Could you check a few things on this model? Use its own coordinates, in mm. A direction names the side the tool comes from. Coordinates: 2 decimals unless noted, no trailing zeros. Loops run counter-clockwise (first coordinate to the right, second up) from the corner with the lowest first, then second, coordinate; pieces in that order, holes last.
from build123d import *

# Parameters (mm, degrees)
BOSS_EXTRUDE1_DEPTH = 60
SKETCH2_W           = 10
SKETCH2_H           = 50
CUT_EXTRUDE1_DEPTH  = 25
SKETCH3_W           = 10
SKETCH3_H           = 50
CUT_EXTRUDE2_DEPTH  = 25
FILLET1_R           = 2
SKETCH4_R           = 2
CUT_EXTRUDE3_DEPTH  = 25


with BuildPart() as part:
    # Sketch1 → Boss-Extrude1 (new body)
    with BuildSketch(Plane(origin=(0, 0, 0), x_dir=(1, 0, 0), z_dir=(0, 1, 0))):
        with BuildLine():
            Line((-4.271755912, 52.025339674), (24.498929667, 52.025339674))
            ThreePointArc((24.498929667, 52.025339674), (-8.501070333, 19.025339674), (24.498929667, -13.974660326))
            Line((24.498929667, -13.974660326), (-4.271755912, -13.974660326))
            Line((-4.271755912, -13.974660326), (-4.271755912, -77.974660326))
            Line((-4.271755912, -77.974660326), (-14.271755912, -77.974660326))
            Line((-14.271755912, -77.974660326), (-14.271755912, 52.025339674))
            Line((-14.271755912, 52.025339674), (-4.271755912, 52.025339674))
        make_face()
    extrude(amount=BOSS_EXTRUDE1_DEPTH)

    # Sketch2 → Cut-Extrude1 (cut)
    with BuildSketch(Plane(origin=(0, 60, 0), x_dir=(1, 0, 0), z_dir=(0, 1, 0))):
        with Locations((-9.271755912, -52.974660326)):
            Rectangle(SKETCH2_W, SKETCH2_H)
    extrude(amount=-CUT_EXTRUDE1_DEPTH, mode=Mode.SUBTRACT)

    # Sketch3 → Cut-Extrude2 (cut)
    with BuildSketch(Plane.XZ):
        with Locations((-9.271755912, 52.974660326)):
            Rectangle(SKETCH3_W, SKETCH3_H)
    extrude(amount=-CUT_EXTRUDE2_DEPTH, mode=Mode.SUBTRACT)

    # Fillet1
    fillet1_edges = [part.edges().sort_by_distance(p)[0] for p in [
        (24.498929667, 30, -52.025339674),
        (24.498929667, 30, 13.974660326),
    ]]
    fillet(fillet1_edges, radius=FILLET1_R)

    # Sketch4 → Cut-Extrude3 (cut)
    with BuildSketch(Plane(origin=(0, 35, 0), x_dir=(1, 0, 0), z_dir=(0, 1, 0))):
        with Locations((-9.271755912, -65.474660326)):
            Circle(SKETCH4_R)
    extrude(amount=-CUT_EXTRUDE3_DEPTH, mode=Mode.SUBTRACT)


solid = part.part
1) Imagine slicing it at C-C on z = -35. List the corners of the cut face in (x, y) for me.
2) Will these pins go through, and if not, where does the flat tip stop? pin 1 (8 mm diameter, centred on x = -10, y = 16.5, fed in from +Z); pin 2 (2.5 mm diameter, centred on x = -9.27, z = 65.47, fed in from +Y); pin 3 (5 mm diameter, centred on x = -11.5, z = 44.5, fed in from -Y); pin 4 (1.5 mm diameter, centred on x = 4.5, y = 19, fed in from +Z).
3) Imagine slicing it at B-B on z = 25.5. List the corners of the cut face in (x, y) for me, plus the area to 3 significant figures.
4) If I drill on L1, parallel to Y at x = -11.5, z = 37; L2, parallel to Z at x = 9.25, y = 4; L3, parallel to Z at x = -3, y = 26, over which ranges is the centre line in solid material (lowest first)?
5) For faces 1 (the flat face through (2, 30, 13.975)), 2 (the flat face through (-9, 48, 27.975)), 3 (the flat face through (-9, 25, 53)), which set-ups out of +Z, -Z, +X, -X, +Y, -Y let a thin tool reach every point of the face, with its end or its side?
6) We'd pull the mould along Z, two halves only. Please class faces 4 (the flat face through (-9, 12, 27.975)), 5 (the flat face through (-4.272, 28, 32)), 6 (the cylindrical face through (10.2, 30.42, 12.42)): released by +Z, released by -Z, zero draft, split by the parting line, or undercut.
7) Imagine slicing it at A-A on x = 0. List the corners of the cut face in (y, z) for me.
Solved:
1. outline: (-14.27, 0) - (-4.38, 0) - (-4.38, 60) - (-14.27, 60) - close
2. pin 1: stops at z = 27.97
2. pin 2: passes through
2. pin 3: stops at y = 25
2. pin 4: stops at z = 13.97
3. outline: (-14.27, 0) - (-4.27, 0) - (-4.27, 60) - (-14.27, 60) - close
3. area: 600 mm2
4. L1: y = 25 to 35
4. L2: z = -51.76 to -48.29, 10.24 to 13.71
4. L3: z = -52.03 to -37.27, -0.78 to 13.97
5. face 1: +Z, +X, +Y, -Y
5. face 2: +Z, +X, -X, +Y
5. face 3: +Z, +X, -X, -Y
6. face 4: released by +Z
6. face 5: zero draft
6. face 6: undercut
7. outline: (0, -52.03) - (60, -52.03) - (60, -41.13) - (0, -41.13) - close; (0, 3.08) - (60, 3.08) - (60, 13.97) - (0, 13.97) - close
